Design review of the part built by this model. Coordinates are the model's own, in mm. A direction names the side the tool comes from. Coordinates: 2 decimals unless noted, no trailing zeros. Write each loop counter-clockwise with the first axis right and the second up, starting at its lowest first coordinate (ties: lowest second). Pieces come first, ordered by that corner, then holes. Notation, with made-up numbers: (-5.75, 25.5) - (34.25, 25.5) arc R18 ccw to (34.25, 36.5) - close; hole circle Ø10 at (3, 13). An arc over 180 degrees is marked (long way). Use a Markdown table: item, result.
from build123d import *

# Parameters (mm, degrees)
SKETCH1_W                = 76.2
SKETCH1_H                = 76.2
BOSS_EXTRUDE1_DEPTH      = 6.35
FILLET1_R                = 2.54
SKETCH3_R                = 1.78
CUT_EXTRUDE1_DEPTH       = 7.35
SKETCH4_W                = 63.5
SKETCH4_H                = 63.5
BOSS_EXTRUDE2_DEPTH      = 2.54
FILLET2_R                = 2.54
M4_CLEARANCE_HOLE2_D     = 4.5
M4_CLEARANCE_HOLE2_DEPTH = 13.97
M4_CLEARANCE_HOLE2_TIP   = 1.351936393
SKETCH7_W                = 50.8
SKETCH7_H                = 3.81
CUT_EXTRUDE2_DEPTH       = 5.08
FILLET3_R                = 1.27


with BuildPart() as part:
    # Sketch1 → Boss-Extrude1 (new body)
    with BuildSketch(Plane(origin=(0, 0, 0), x_dir=(1, 0, 0), z_dir=(0, 1, 0))):
        Rectangle(SKETCH1_W, SKETCH1_H)
    extrude(amount=BOSS_EXTRUDE1_DEPTH)

    # Fillet1
    fillet1_edges = [part.edges().sort_by_distance(p)[0] for p in [
        (38.1, 3.175, 38.1),
        (-38.1, 3.175, 38.1),
        (-38.1, 3.175, -38.1),
        (38.1, 3.175, -38.1),
    ]]
    fillet(fillet1_edges, radius=FILLET1_R)

    # Sketch3 → Cut-Extrude1 (cut, through all)
    with BuildSketch(Plane(origin=(0, 6.35, 0), x_dir=(1, 0, 0), z_dir=(0, 1, 0))):
        Circle(SKETCH3_R)
    extrude(amount=-CUT_EXTRUDE1_DEPTH, mode=Mode.SUBTRACT)

    # Sketch4 → Boss-Extrude2 (add)
    with BuildSketch(Plane.XZ):
        Rectangle(SKETCH4_W, SKETCH4_H)
    extrude(amount=BOSS_EXTRUDE2_DEPTH)

    # Fillet2
    fillet2_edges = [part.edges().sort_by_distance(p)[0] for p in [
        (-31.75, -1.27, 31.75),
        (-31.75, -1.27, -31.75),
        (31.75, -1.27, -31.75),
        (31.75, -1.27, 31.75),
    ]]
    fillet(fillet2_edges, radius=FILLET2_R)

    # M4 Clearance Hole2
    with Locations(Plane.XZ.offset(2.54)):
        with Locations((-34.181051224, 34.181051224), (-34.181051224, -34.181051224), (34.181051224, -34.181051224), (34.181051224, 34.181051224)):
            Hole(M4_CLEARANCE_HOLE2_D / 2, depth=M4_CLEARANCE_HOLE2_DEPTH)
            with Locations((0, 0, -(M4_CLEARANCE_HOLE2_DEPTH + M4_CLEARANCE_HOLE2_TIP / 2))):  # 118° drill point
                Cone(0, M4_CLEARANCE_HOLE2_D / 2, M4_CLEARANCE_HOLE2_TIP, mode=Mode.SUBTRACT)

    # Sketch7 → Cut-Extrude2 (cut)
    with BuildSketch(Plane(origin=(0, -2.54, 0), x_dir=(-1, 0, 0), z_dir=(0, -1, 0))):
        with Locations((0, 27.94)):
            Rectangle(SKETCH7_W, SKETCH7_H)
        with Locations((0, -27.94)):
            Rectangle(SKETCH7_W, SKETCH7_H)
    extrude(amount=-CUT_EXTRUDE2_DEPTH, mode=Mode.SUBTRACT)

    # Fillet3
    fillet3_edges = [part.edges().sort_by_distance(p)[0] for p in [
        (25.4, 0, -26.035),
        (25.4, 0, -29.845),
        (-25.4, 0, -29.845),
        (-25.4, 0, -26.035),
        (25.4, 0, 29.845),
        (25.4, 0, 26.035),
        (-25.4, 0, 26.035),
        (-25.4, 0, 29.845),
    ]]
    fillet(fillet3_edges, radius=FILLET3_R)


solid = part.part
(1) For pin 1 (5 mm diameter, centred on x = 34.18, z = -34.18, fed in from +Y); pin 2 (0.8 mm diameter, centred on y = -1, z = -1.5, fed in from +X); pin 3 (1.5 mm diameter, centred on x = 9, y = -1, fed in from -Z); pin 4 (5 mm diameter, centred on x = -34.18, z = -34.18, fed in from -Y), all flat-tipped, find the tip position at first contact; note any pin that passes through.
Determined:
| item | result |
|---|---|
| pin 1 | y = 6.35 |
| pin 2 | x = 31.75 |
| pin 3 | z = -31.75 |
| pin 4 | y = 0 |
(2) Draft analysis for pull direction Z (two halves, no side actions). For faces 1 (the flat face through (38.1, 3, 0)), 2 (the flat face through (0, 0, 0)), 3 (the cylindrical face through (30.986, -1.288, 31.026)), 4 (the flat face through (0, 0, -29.845)), state which applies: +Z half, -Z half, draft (parallel to the pull), parting line (faces both ways), or undercut.
Determined:
| item | result |
|---|---|
| face 1 | draft |
| face 2 | undercut |
| face 3 | +Z half |
| face 4 | undercut |
(3) For L1, parallel to Z at x = -3, y = -1.25 (3 decimals); L2, parallel to Z at x = -15, y = 1.5 (3 decimals); L3, parallel to Z at x = 0, y = 2.5 (3 decimals), list the stretches that pass through material, from the lowest coordinate up. Write a range as from..to.
Determined:
| item | result |
|---|---|
| L1 | -31.75..-29.845, -26.035..26.035, 29.845..31.75 |
| L2 | -38.1..-29.845, -26.035..26.035, 29.845..38.1 |
| L3 | -38.1..-29.845, -26.035..-1.78, 1.78..26.035, 29.845..38.1 |
(4) Take a section at C-C on z = 0. Write out the cut boundary in (x, y), and give its area (3 significant figures).
Determined:
| item | result |
|---|---|
| outline | (-38.1, 0) - (-31.75, 0) - (-31.75, -2.54) - (31.75, -2.54) - (31.75, 0) - (38.1, 0) - (38.1, 6.35) - (1.78, 6.35) - (1.78, 0) - (-1.78, 0) - (-1.78, 6.35) - (-38.1, 6.35) - close |
| area | 623 mm2 |
(5) Take a section at A-A on z = -22. Write out the cut boundary in (x, y), and give its area (3 significant figures).
Determined:
| item | result |
|---|---|
| outline | (-38.1, 0) - (-31.75, 0) - (-31.75, -2.54) - (31.75, -2.54) - (31.75, 0) - (38.1, 0) - (38.1, 6.35) - (-38.1, 6.35) - close |
| area | 645 mm2 |
(6) Take a section at B-B on x = -3. Write out the cut boundary in (y, z) (3 decimals).
Determined:
| item | result |
|---|---|
| outline | (-2.54, -31.75) - (0, -31.75) - (0, -38.1) - (6.35, -38.1) - (6.35, 38.1) - (0, 38.1) - (0, 31.75) - (-2.54, 31.75) - (-2.54, 29.845) - (2.54, 29.845) - (2.54, 26.035) - (-2.54, 26.035) - (-2.54, -26.035) - (2.54, -26.035) - (2.54, -29.845) - (-2.54, -29.845) - close |
(7) Machinability: for faces 5 (the flat face through (0, -1, 31.75)), 6 (the flat face through (-31.75, -1, 0)), 7 (the flat face through (31.75, -1, 0)), 8 (the cylindrical face through (-37.376, 3.219, 37.336)), 9 (the flat face through (0, 0, 26.035)), which of the approach directions +Z, -Z, +X, -X, +Y, -Y give a long, thin tool a straight path to every point of the face, cutting with its end or side? Answer none if there is none.
Determined:
| item | result |
|---|---|
| face 5 | +Z, +X, -X, -Y |
| face 6 | +Z, -Z, -X, -Y |
| face 7 | +Z, -Z, +X, -Y |
| face 8 | +Z, -X, +Y, -Y |
| face 9 | -Y |
